Input: part model. Units: mm. Frame: model coordinates. A direction names the side the tool comes from. Give positions to 0.01 mm unless a question says otherwise; leave off trailing zeros. Order: outer loops, then holes, each group sorted by start corner. A loop starts at its lowest first (then second) coordinate and runs counter-clockwise, first axis right, second up. Notation, with made-up numbers: (-16, 47) - (2, 47) arc R3 ccw to (2, 51) - close; hole circle Ø7 at (66.25, 42.5). An arc over 180 degrees is marked (long way). Answer in a Markdown table with one row per item. Add a question column.
1. Section query B-B on y = 6.75. Return loops of the section in (x, z).
2. Section query D-D on y = 10.5. Return loops of the section in (x, z).
3. Contact query for flat-ended pins moving along their axis: pin 1 (6 mm diameter, centred on y = 7.5, z = 2, fed in from -X); pin 2 (3 mm diameter, centred on x = 17, z = -3.5, fed in from +Y). Output: stop coordinate, or through.
4. Mould query, pull axis Z, two halves, no side actions, for faces 3 (the face through (-6, 1, 0)), 4 (the face through (50.889, 0.663, 0.084)), 5 (the face through (50.78, 6.11, 0.08)), 6 (the face through (-1.947, 0.783, -2.539)). Classes: released by +Z, released by -Z, zero draft, split by the parting line, or undercut.
5. Access query for faces 1 (the face through (22, 0, 0)), 2 (the face through (50, 5.7, 0.1)). Directions: +Z, -Z, +X, -X, +Y, -Y. A direction counts if a zero-diameter tool reaches every point of the face in a straight line with its end or side. Return the directions, or none.
6. Section query C-C on x = 31.5. Return loops of the section in (y, z), and give its area (4 significant figures).
7. Section query A-A on z = 0. Return loops of the section in (x, y).
8. Ray query, line 1 (Y direction, x = 40, z = -4); line 2 (X direction, y = 10.25, z = -1.5); line 3 (X direction, y = 0.9, z = 0). Return the intervals inside material, ascending. Write a range as [from, to].
```python
from build123d import *

# Parameters (mm, degrees)
SKETCH1_R                    = 3.2
BASE_FLANGE1_DEPTH           = 1.5875
EDGE_FLANGE1_STRIP_W         = 7.8232
EDGE_FLANGE1_STRIP_H         = 1.5875
EDGE_FLANGE1_STRIP_CUT_DEPTH = 12
EDGE_FLANGE1_DEPTH           = 12
HOLE1_START                  = 50
HOLE1_OUTLINE_R              = 1.8288
HOLE1_DEPTH                  = 1.5875
FILLET1_RADIUS               = 6
FILLET1_LENGTH               = 1.5875


# Read off the part's stored shape, not the designer's step: Hole1
# Sheet-metal steps are written as plain solids
with BuildPart() as part:
    # Sketch1 → Base-Flange1 (new body)
    with BuildSketch(Plane(origin=(0, 0, 0), x_dir=(1, 0, 0), z_dir=(0, 1, 0))):
        with BuildLine():
            Line((0, 6), (50, 6))
            Line((50, 6), (50, -6))
            Line((50, -6), (0, -6))
            ThreePointArc((0, -6), (-6, 0), (0, 6))
        make_face()
        with Locations(Location((0, 0, 0), (0, 0, 270))):
            Circle(SKETCH1_R, mode=Mode.SUBTRACT)
    extrude(amount=BASE_FLANGE1_DEPTH)

    # Edge-Flange1 strip (across the edge) → Edge-Flange1 strip cut (cut)
    with BuildSketch(Plane(origin=(50, 1.5875, 6), x_dir=(-1, 0, 0), z_dir=(0, 0, -1))):
        with Locations((-3.175, -0.79375)):
            Rectangle(EDGE_FLANGE1_STRIP_W, EDGE_FLANGE1_STRIP_H)
    extrude(amount=EDGE_FLANGE1_STRIP_CUT_DEPTH, mode=Mode.SUBTRACT)

    # Edge-Flange1 section (across the edge) → Edge-Flange1 (add)
    with BuildSketch(Plane(origin=(50, 1.5875, 6), x_dir=(-1, 0, 0), z_dir=(0, 0, -1))):
        with BuildLine():
            Line((-1.5875, 0.7366), (-1.5875, 12.7))
            Line((-1.5875, 12.7), (0, 12.7))
            Line((0, 12.7), (0, 0.7366))
            ThreePointArc((0, 0.7366), (0.215745145, 0.215745145), (0.7366, 0))
            Line((0.7366, 0), (0.7366, -1.5875))
            ThreePointArc((0.7366, -1.5875), (-0.90678687, -0.90678687), (-1.5875, 0.7366))
        make_face()
    extrude(amount=EDGE_FLANGE1_DEPTH)

    # Hole1 outline → Hole1 (cut)
    with BuildSketch(Plane.YZ.offset(HOLE1_START)):
        with Locations((7.9375, 0)):
            Circle(HOLE1_OUTLINE_R)
    extrude(amount=HOLE1_DEPTH, mode=Mode.SUBTRACT)

    # Fillet1: full round fillet: the end face becomes a half cylinder, R = half its width
    fillet1_face = Plane((50.79375, 14.2875, 0), x_dir=(1, 0, 0), z_dir=(0, 1, 0))  # on the end face: x along it, z out of the body
    fillet1_slab = fillet1_face.offset(-FILLET1_RADIUS / 2) * Box(FILLET1_LENGTH, 2 * FILLET1_RADIUS, FILLET1_RADIUS, mode=Mode.PRIVATE)  # the body's end, R deep
    fillet1_round = Plane((50.79375, 8.2875, 0), x_dir=(0, 1, 0), z_dir=(1, 0, 0)) * Cylinder(FILLET1_RADIUS, FILLET1_LENGTH, mode=Mode.PRIVATE)  # its axis R under the face
    add(fillet1_slab - fillet1_round, mode=Mode.SUBTRACT)


solid = part.part
```
Answer:
| question | item | result |
|---|---|---|
| 1 | outline | (50, -6) - (51.59, -6) - (51.59, -1.39) - (50, -1.39) - close; (50, 1.39) - (51.59, 1.39) - (51.59, 6) - (50, 6) - close |
| 2 | outline | (50, -5.58) - (51.59, -5.58) - (51.59, 5.58) - (50, 5.58) - close |
| 3 | pin 1 | stops at x = 50 |
| 3 | pin 2 | stops at y = 1.59 |
| 4 | face 3 | split by the parting line |
| 4 | face 4 | zero draft |
| 4 | face 5 | undercut |
| 4 | face 6 | undercut |
| 5 | face 1 | +Z, -Z, +X, -X, -Y |
| 5 | face 2 | +Z, -Z, -X, +Y |
| 6 | outline | (0, -6) - (1.59, -6) - (1.59, 6) - (0, 6) - close |
| 6 | area | 19.05 mm² |
| 7 | outline | (-6, 0) - (-3.2, 0) - (-3.2, 1.59) - (-6, 1.59) - close; (3.2, 0) - (49.26, 0) arc R2.32 ccw to (51.59, 2.32) - (51.59, 6.11) - (50, 6.11) - (50, 2.32) arc R0.74 cw to (49.26, 1.59) - (3.2, 1.59) - close; (50, 9.77) - (51.59, 9.77) - (51.59, 14.29) - (50, 14.29) - close |
| 8 | line 1 | y = [0, 1.59] |
| 8 | line 2 | x = [50, 51.59] |
| 8 | line 3 | x = [-6, -3.2], [3.2, 51.1] |
